Input: part model. Units: mm. Frame: model coordinates. A direction names the side the tool comes from. Coordinates: 2 decimals unless noted, no trailing zeros. Write each loop counter-clockwise with the first axis right and the second up, starting at its lowest first coordinate (ties: lowest second). Pieces come first, ordered by that corner, then holes. Notation, with made-up numbers: (20, 78) -> (75, 78) arc R23 ccw to (75, 106) -> close; hole circle Ø11 at (79.5, 70). An arc over 180 degrees is marked (long way). One line per question, with ' | ' between items. Start each with the question number.
Autodesk Inventor part; units mm, degrees
ref_plane "YZ Plane" through (0, 0, 0) normal (1, 0, 0) x (0, 1, 0)
ref_plane "XZ Plane" through (0, 0, 0) normal (0, 1, 0) x (-1, 0, 0)
ref_plane "XY Plane" through (0, 0, 0) normal (0, 0, 1) x (1, 0, 0)
sketch "Náčrt1" plane through (0, 0, 0) normal (0, 0, 1) x (1, 0, 0)
  line L0 (-42.48, 0) -> (7.08, 0)
  line L1 (0, 37.68) -> (0, -6.28)
  line L2 (-35.4, 0) -> (0, 0)
  line L3 (-35.4, 0) -> (-35.4, 30)
  line L4 (-35.4, 30) -> (-33.2, 30)
  line L5 (-33.2, 30) -> (-33.2, 31.4)
  line L6 (-33.2, 31.4) -> (-28.2, 31.4)
  line L7 (-28.2, 31.4) -> (-28.2, 30)
  line L8 (-28.2, 30) -> (-26, 30)
  line L9 (-26, 30) -> (-26, 29.05)
  line L10 (-26, 29.05) -> (0, 29.05)
  line L11 (0, 29.05) -> (0, 0)
  point P0 (0, 0)
  point P1 (0, 29.05)
  dimension "d1" = 29.05
  dimension "d2" = 30
  dimension "d3" = 31.4
  dimension "d4" = 35.4
  dimension "d5" = 2.2
  dimension "d6" = 2.2
  dimension "d7" = 5
revolve "Rotace1" add sketch "Náčrt1" angle 360 about axis through (0, 0, 0) along (1, 0, 0)
properties part number "prop_meter"
1) Access query for faces 1 (the face through (-33.2, 30.1, -2.2)), 2 (the face through (-35.4, 0, 0)), 3 (the face through (-27.08, -29.97, 1.32)). Directions: +Z, -Z, +X, -X, +Y, -Y. A direction counts if a zero-diameter tool reaches every point of the face in a straight line with its end or side. Return the directions, or none.
2) First-contact query: P1, Ø4, axis at x = -7.5, y = -10, coming from the +Z side; P2, Ø3, axis at x = -14.5, y = -7, coming from the +Z side; P3, Ø5, axis at x = -22, z = 17.5, coming from the -Y side. Flat tips, straight axial feed; report the tip coordinate or a pass-through.
3) Section C-C, the plane x = -16. Return loops of the section in (y, z).
4) Ray query, line 1 (X direction, y = -27.5, z = 13.5); line 2 (Y direction, x = -23, z = -23); line 3 (Y direction, x = -23.5, z = 7). Return the intervals inside material, ascending.
5) Section A-A, the plane y = 0. Return loops of the section in (x, z).
6) Section D-D, the plane x = -31. Return loops of the section in (y, z).
Answer block:
1) face 1: -X | face 2: +Z, -Z, -X, +Y, -Y | face 3: +X
2) P1: stops at z = 27.93 | P2: stops at z = 28.52 | P3: stops at y = -24.88
3) outline: circle Ø58.1 at (0, 0)
4) line 1: x = -33.2 to -28.2 | line 2: y = -17.75 to 17.75 | line 3: y = -28.19 to 28.19
5) outline: (-35.4, -30) -> (-33.2, -30) -> (-33.2, -31.4) -> (-28.2, -31.4) -> (-28.2, -30) -> (-26, -30) -> (-26, -29.05) -> (0, -29.05) -> (0, 29.05) -> (-26, 29.05) -> (-26, 30) -> (-28.2, 30) -> (-28.2, 31.4) -> (-33.2, 31.4) -> (-33.2, 30) -> (-35.4, 30) -> close
6) outline: circle Ø62.8 at (0, 0)
